Geometry: final body of the model. Coordinates: model frame, mm. Give positions to 0.01 mm unless a question says otherwise; leave off trailing zeros. Write each loop counter-clockwise with the first axis right and the second up, starting at its lowest first coordinate (ties: lowest second). Pieces come first, ordered by that corner, then holes.
Q1. Line query: line 1 (Z direction, x = 0, y = -4.2); line 2 (X direction, y = -6.5, z = 18.5); line 3 (Z direction, x = 0, y = -2.1). Output: solid intervals per line, ascending.
Q2. Section C-C (z = 50.5). Return the cut outline in (x, y).
Q3. Section B-B (y = -4.75). Return the cut outline in (x, z).
Q4. Section D-D (x = -14). Return the cut outline in (y, z), plus the area to 3 significant figures.
Q5. Mould query, pull axis Z, two halves, no side actions, for faces 1 (the flat face through (-11, 0, 27)), 2 (the cylindrical face through (18.1, -3.51, 54.46)), 3 (the cylindrical face through (0.224, -6.098, -15.829)), 4 (the cylindrical face through (-1.432, -3.458, 30.222)). Classes: +Z half, -Z half, draft (parallel to the pull), parting line (faces both ways), or undercut.
Q6. Section A-A (x = 0). Return the cut outline in (y, z).
from build123d import *

# Parameters (mm, degrees)
F0_R     = 11
F1_DEPTH = 7
F2_R     = 3
F3_R     = 0.5


with BuildPart() as f1:
    # F0 (on Front) → F1 (new body)
    with BuildSketch(Plane.XZ):
        Polygon((19, 55.315645), (0, 55.315645), (-19, 55.315645), (-19, -16.684355), (0, -16.684355), (19, -16.684355), align=None)
        with Locations((0, 19.315645)):
            Circle(F0_R, mode=Mode.SUBTRACT)
    extrude(amount=F1_DEPTH)

    # F2
    f2_edges = [f1.edges().sort_by_distance(p)[0] for p in [
        (0, -7, 55.315645),
        (0, 0, 55.315645),
        (19, 0, 19.315645),
        (-19, -7, 19.315645),
        (19, -7, 19.315645),
        (0, -7, -16.684355),
        (0, 0, -16.684355),
        (19, -3.5, -16.684355),
        (-19, -3.5, -16.684355),
        (-19, 0, 19.315645),
        (-19, -3.5, 55.315645),
        (19, -3.5, 55.315645),
    ]]
    fillet(f2_edges, radius=F2_R)

    # F3
    f3_edges = [f1.edges().sort_by_distance(p)[0] for p in [
        (-11, -7, 19.315645),
        (-11, 0, 19.315645),
    ]]
    fillet(f3_edges, radius=F3_R)


solid = f1.part
Computed:
1. line 1: z = -16.68 to 8.32, 30.32 to 55.31
1. line 2: x = -17.66 to -10.97, 10.97 to 17.66
1. line 3: z = -16.55 to 8.32, 30.32 to 55.18
2. outline: (-19, -4) arc R3 ccw to (-16, -7) - (16, -7) arc R3 ccw to (19, -4) - (19, -3) arc R3 ccw to (16, 0) - (-16, 0) arc R3 ccw to (-19, -3) - close
3. outline: (-18.9, -13.68) arc R2.9 ccw to (-16, -16.59) - (16, -16.59) arc R2.9 ccw to (18.9, -13.68) - (18.9, 52.32) arc R2.9 ccw to (16, 55.22) - (-16, 55.22) arc R2.9 ccw to (-18.9, 52.32) - close; hole circle Ø22 at (0, 19.32)
4. outline: (-7, -13.68) arc R3 ccw to (-4, -16.68) - (-3, -16.68) arc R3 ccw to (0, -13.68) - (0, 52.32) arc R3 ccw to (-3, 55.32) - (-4, 55.32) arc R3 ccw to (-7, 52.32) - close
4. area: 496 mm2
5. face 1: draft
5. face 2: +Z half
5. face 3: -Z half
5. face 4: undercut
6. outline: (-7, -13.68) arc R3 ccw to (-4, -16.68) - (-3, -16.68) arc R3 ccw to (0, -13.68) - (0, 7.82) arc R0.5 ccw to (-0.5, 8.32) - (-6.5, 8.32) arc R0.5 ccw to (-7, 7.82) - close; (-7, 30.82) arc R0.5 ccw to (-6.5, 30.32) - (-0.5, 30.32) arc R0.5 ccw to (0, 30.82) - (0, 52.32) arc R3 ccw to (-3, 55.32) - (-4, 55.32) arc R3 ccw to (-7, 52.32) - close
